Could you check a few things on this model? Use its own coordinates, in mm. Face numbers are marked on the shaded views. A direction names the side the tool comes from. Coordinates: 2 decimals unless noted, no trailing zeros. Loops run counter-clockwise (first coordinate to the right, second up) from the corner with the lowest first, then second, coordinate; pieces in that order, holes last.
Autodesk Inventor part; units mm, degrees
ref_plane "YZ Plane" through (0, 0, 0) normal (1, 0, 0) x (0, 1, 0)
ref_plane "XZ Plane" through (0, 0, 0) normal (0, 1, 0) x (-1, 0, 0)
ref_plane "XY Plane" through (0, 0, 0) normal (0, 0, 1) x (1, 0, 0)
sketch "Sketch1" plane through (0, 0, 0) normal (0, 1, 0) x (-1, 0, 0)
  line L0 (10, 20) -> (-10, 20)
  line L1 (-10, 20) -> (-10, -20)
  line L2 (-10, -20) -> (10, -20)
  line L3 (10, -20) -> (10, 20)
  line L4 (10, 20) -> (-10, -20) construction
  line L5 (-10, 20) -> (10, -20) construction
  point P0 (0, 0)
  dimension "d2" = 20
  dimension "d3" = 40
extrude "Extrusion1" add sketch "Sketch1" along normal mid plane 5
sketch "Sketch2" plane through (0, 2.5, 0) normal (0, 1, 0) x (1, 0, 0)
  line L0 (10, -4) -> (-10, -4)
  line L1 (-10, -4) -> (-10, -7)
  line L2 (-10, -7) -> (10, -7)
  line L3 (10, -7) -> (10, -4)
  line L4 (10, -17) -> (-10, -17)
  line L5 (-10, -17) -> (-10, -20)
  line L6 (-10, -20) -> (10, -20)
  line L7 (10, -20) -> (10, -17)
  line L8 (10, -20) -> (10, 20)
  line L9 (-10, 20) -> (-10, -20)
  line L10 (10, 20) -> (-10, 20)
  line L11 (-10, -20) -> (10, -20)
  point P0 (0, 0)
  dimension "d4" = 3
  dimension "d5" = 3
  dimension "d6" = 10
extrude "Extrusion2" add sketch "Sketch2" along normal blind 3 contours L3 L2 L1 L0 | L7 L6 L5 L4
sketch "Sketch3" plane through (0, 2.5, 0) normal (0, 1, 0) x (1, 0, 0)
  line L0 (10, -7) -> (-10, -7)
  line L1 (-10, -7) -> (-10, -17)
  line L2 (-10, -17) -> (10, -17)
  line L3 (10, -17) -> (10, -7)
  line L4 (10, -17) -> (-10, -17)
  point P0 (0, 0)
  point P1 (0, -12)
  point P2 (-10, -12)
  point P3 (0, -17)
hole "Hole1" at (0, 2.5, 12) direction (0, -1, 0) diameter 4.305 end through all
sketch "Sketch4" plane through (0, -2.5, 0) normal (0, -1, 0) x (1, 0, 0)
  circle A0 centre (0, -4.677) radius 3.9688
  circle A1 centre (0, 12) radius 2.1525
  point P0 (0, 0)
  dimension "d16" = 7.9375
  dimension "d17" = 16.677
extrude "Extrusion3" add sketch "Sketch4" along normal blind 4 contours A0
sketch "Sketch6" plane through (0, -2.5, 0) normal (0, -1, 0) x (1, 0, 0)
  circle A0 centre (7.5, -17.5) radius 1
  circle A1 centre (-7.5, -17.5) radius 1
  line L0 (-10, -20) -> (10, -20)
  line L1 (10, -20) -> (10, 20)
  line L2 (-10, 20) -> (-10, -20)
  point P0 (0, 0)
  point P1 (-8, -17.5)
  point P2 (8, -17.5)
  point P3 (10, -15.5)
  point P4 (10, 15.5)
  point P5 (-10, 15.5)
  point P6 (-10, -15.5)
  dimension "d28" = 2
  dimension "d29" = 2
  dimension "d30" = 2.5
  dimension "d31" = 2.5
  dimension "d32" = 2.5
extrude "Extrusion5" cut sketch "Sketch6" against normal through all
sketch "Sketch8" plane through (0, -2.5, 0) normal (0, -1, 0) x (1, 0, 0)
  line L0 (10, 20) -> (10, 17)
  line L1 (10, 17) -> (-10, 17)
  line L2 (10, 20) -> (-10, 20)
  line L3 (-10, 20) -> (-10, 17)
  line L4 (-10, 17) -> (10, 17)
  line L5 (10, 17) -> (10, 20)
  point P0 (0, 0)
extrude "Extrusion6" add sketch "Sketch8" along normal blind 5
sketch "Sketch9" plane through (0, -7.5, 0) normal (0, -1, 0) x (1, 0, 0)
  circle A0 centre (8, 18.5) radius 1
  circle A1 centre (-8, 18.5) radius 1
  line L0 (10, 17) -> (10, 20)
  line L1 (10, 20) -> (-10, 20)
  line L2 (-10, 20) -> (-10, 17)
  point P0 (0, 0)
  dimension "d38" = 2
  dimension "d39" = 2
  dimension "d40" = 2
  dimension "d41" = 1.5
  dimension "d42" = 2
extrude "Extrusion7" cut sketch "Sketch9" against normal blind 3
fillet "Fillet2" radius 2 4 edges at (-10, -1, 20) (-10, 0, -20) (10, 0, -20) (10, -1, 20)
equation "\"d5\" = d4"
equation "\"d31\" = d30"
equation "\"d32\" = d30"
equation "\"d42\" = d40"
properties part number "PinionHolder"
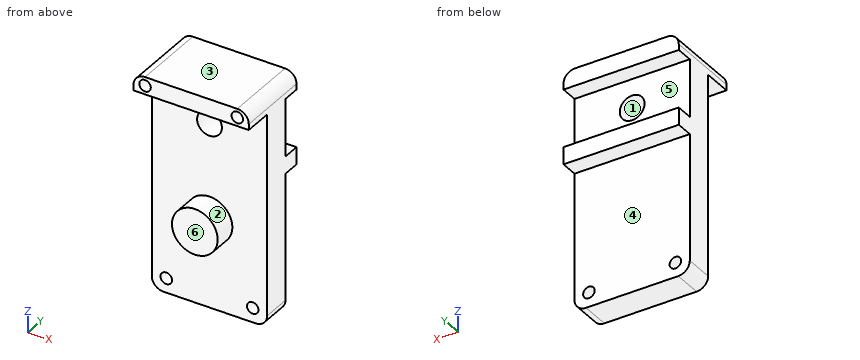
(1) Imagine slicing it at B-B, the plane y = 3.5. Write out the boundary of the cut face in (x, z).
Answers:
outline: (-10, 4) - (10, 4) - (10, 7) - (-10, 7) - close; (-10, 17) - (10, 17) - (10, 18) arc R2 ccw to (8, 20) - (-8, 20) arc R2 ccw to (-10, 18) - close
(2) Which directions (+Z, -Z, +X, -X, +Y, -Y) give clear straight access to the entire face, cutting with the end or side of a thin tool? Please do the marked faces 4, 5 and 6.
Answers:
face 4: -Z, +X, -X, +Y
face 5: +X, -X, +Y
face 6: -Z, +X, -X, -Y
(3) Imagine slicing it at A-A, the plane z = -17.5. Write out the boundary of the cut face in (x, y), and give its area (3 significant figures).
Answers:
outline: (-10, -2.5) - (-8.5, -2.5) - (-8.5, 2.5) - (-10, 2.5) - close; (-6.5, -2.5) - (6.5, -2.5) - (6.5, 2.5) - (-6.5, 2.5) - close; (8.5, -2.5) - (10, -2.5) - (10, 2.5) - (8.5, 2.5) - close
area: 80.0 mm2
(4) We'd pull the mould along X, two halves only. Please class the marked faces 1, 2 and 3: +X half, -X half, draft (parallel to the pull), parting line (faces both ways), or undercut.
Answers:
face 1: undercut
face 2: parting line
face 3: draft
(5) For pin 1 (1.5 mm diameter, centred on x = 4.5, z = -3, fed in from -Y); pin 2 (2.5 mm diameter, centred on x = 7.5, z = -17.5, fed in from +Y); pin 3 (2.5 mm diameter, centred on x = 1, y = 4, fed in from -Z); pin 4 (2.5 mm diameter, centred on x = 0, z = 12, fed in from -Y), each with a flat end and sliding along its axis, tell me the tip position at first contact or that it passes through.
Answers:
pin 1: stops at y = -2.5
pin 2: stops at y = 2.5
pin 3: stops at z = 4
pin 4: passes through
(6) Imagine slicing it at C-C, the plane x = 0. Write out the boundary of the cut face in (y, z), and give its area (3 significant figures).
Answers:
outline: (-7.5, 17) - (-2.5, 17) - (-2.5, 14.15) - (2.5, 14.15) - (2.5, 17) - (5.5, 17) - (5.5, 20) - (-7.5, 20) - close; (-6.5, -8.65) - (-2.5, -8.65) - (-2.5, -20) - (2.5, -20) - (2.5, 4) - (5.5, 4) - (5.5, 7) - (2.5, 7) - (2.5, 9.85) - (-2.5, 9.85) - (-2.5, -0.71) - (-6.5, -0.71) - close
area: 243 mm2
(7) I need wall thicknesses on probe 1 along Z at (x, y) = (0, 1.4); probe 2 along Z at (x, y) = (-5.25, 4); probe 3 along X at (y, z) = (0.05, 12). Which ranges of each line are inside material? Lowest first, please.
Answers:
probe 1: z = -20 to 9.85, 14.15 to 20
probe 2: z = 4 to 7, 17 to 20
probe 3: x = -10 to -2.15, 2.15 to 10
(8) Imagine slicing it at D-D, the plane z = 12. Write out the boundary of the cut face in (x, y).
Answers:
outline: (-10, -2.5) - (-2.15, -2.5) - (-2.15, 2.5) - (-10, 2.5) - close; (2.15, -2.5) - (10, -2.5) - (10, 2.5) - (2.15, 2.5) - close
